Verification items for the finished model (mm, model axes). A direction names the side the tool comes from. Coordinates: 2 decimals unless noted, no trailing zeros. Loops run counter-clockwise (first coordinate to the right, second up) from the corner with the lowest first, then second, coordinate; pieces in that order, holes last. Notation, with made-up numbers: (48.5, -7.75) -> (55.5, -7.75) arc R15 cw to (55.5, 14.25) -> close; hole circle Ø5 at (69.5, 57). An arc over 180 degrees is marked (long way). Answer as a JSON object with one key per item and string values. Group by question number.
Q1. Gauge pin test, flat ends, axial feed: pin 1 Ø1.5 at (x, y) = (11, 10.5) entering from -Z; pin 2 Ø1.5 at (x, z) = (8, -28.5) entering from -Y; pin 3 Ø1.5 at (y, z) = (7.5, -29) entering from +X. Record the tip position at first contact, or that the pin passes through.
Q2. Release check for a two-part mould opening along X. For faces 1 (the cylindrical face through (-0.53, 13.82, -28.87)), 2 (the flat face through (-1, 0, 0)), 3 (the cylindrical face through (-0.53, -13.82, -28.74)), 4 (the flat face through (37.744, 0, -29)) record: released by +X, released by -X, zero draft, split by the parting line, or undercut.
Q3. Cross-section at D-D on y = 15. Record the boundary of the cut face in (x, z) (3 decimals), and give its area (3 significant figures).
Q4. Cross-section at B-B on y = 5. Record the boundary of the cut face in (x, z) (3 decimals).
Q5. Cross-section at A-A on x = 18.5. Record the boundary of the cut face in (y, z).
Q6. Set-up check for faces 5 (the flat face through (-3, -18, -31.75)), 6 (the flat face through (34.2, -6.47, -0.73)), 7 (the flat face through (-1, 16.764, -13)), 8 (the flat face through (-33.096, 0, -1)): record each of +Z, -Z, +X, -X, +Y, -Y from which the full face is reachable in a straight line by a thin tool's end or side.
Q7. Scan lines: L1, parallel to Y at x = 14, z = -24; L2, parallel to X at y = 0, z = -24; L3, parallel to Z at x = -35, y = 9. Record each from-to range of solid material in increasing order.
Q8. Cross-section at C-C on z = -6.5. Record the boundary of the cut face in (x, y).
```python
from build123d import *

# Parameters (mm, degrees)
F0_W      = 79.0448
F0_H      = 37.211
F0_W_2    = 75.438
F0_H_2    = 33.528
F1_DEPTH  = 31.75
F0_W_3    = 29.9212
F0_H_3    = 22.098
F2_DEPTH  = 1.4732
F5_DEPTH  = 35.3695
F7_DEPTH  = 77.2414
F8_W      = 1.778
F8_H      = 2.9464
F9_DEPTH  = 37.211
F10_W     = 1.778
F10_H     = 2.9464
F11_DEPTH = 75.4888


with BuildPart() as f1:
    # F0 (on Top) → F1 (new body)
    with BuildSketch(Plane.XY):
        Rectangle(F0_W, F0_H)
        Rectangle(F0_W_2, F0_H_2, mode=Mode.SUBTRACT)
    extrude(amount=-F1_DEPTH)

    # F0 (on Top) → F2 (join)
    with BuildSketch(Plane.XY):
        Rectangle(F0_W_2, F0_H_2)
        with Locations((-18.1356, 0)):
            Rectangle(F0_W_3, F0_H_3, mode=Mode.SUBTRACT)
        Polygon((9.525, 9.0805), (36.449, 9.0805), (36.449, -3.07601), (31.877, -9.9695), (14.097, -9.9695), (9.525, -3.07601), align=None, mode=Mode.SUBTRACT)
    extrude(amount=-F2_DEPTH)

    # F4 (on face) → F5 (join, through all)
    with BuildSketch(Plane.XZ.offset(18.6055)):
        with BuildLine():
            Line((-37.719, -25.8572), (-37.719, -31.75))
            ThreePointArc((-37.719, -31.75), (-34.7726, -28.8036), (-37.719, -25.8572))
        make_face()
        with BuildLine():
            Line((37.719, -31.75), (37.719, -25.8572))
            ThreePointArc((37.719, -25.8572), (34.7726, -28.8036), (37.719, -31.75))
        make_face()
    extrude(amount=-F5_DEPTH)

    # F6 (on face) → F7 (join, through all)
    with BuildSketch(Plane(origin=(-39.5224, 0, 0), x_dir=(0, -1, 0), z_dir=(-1, 0, 0))):
        with BuildLine():
            Line((-16.764, -25.8572), (-16.764, -31.75))
            ThreePointArc((-16.764, -31.75), (-13.8176, -28.8036), (-16.764, -25.8572))
        make_face()
        with BuildLine():
            Line((16.764, -31.75), (16.764, -25.8572))
            ThreePointArc((16.764, -25.8572), (13.8176, -28.8036), (16.764, -31.75))
        make_face()
    extrude(amount=-F7_DEPTH)

    # F8 (on face) → F9 (cut, through all)
    with BuildSketch(Plane.XZ.offset(18.6055)):
        with Locations((-38.6334, -28.8036)):
            Rectangle(F8_W, F8_H)
        with Locations((38.6334, -28.8036)):
            Rectangle(F8_W, F8_H)
    extrude(amount=-F9_DEPTH, mode=Mode.SUBTRACT)

    # F10 (on face) → F11 (cut, through all)
    with BuildSketch(Plane(origin=(-37.7444, 0, 0), x_dir=(0, -1, 0), z_dir=(-1, 0, 0))):
        with Locations((-17.7165, -28.8036)):
            Rectangle(F10_W, F10_H)
        with Locations((17.7165, -28.8036)):
            Rectangle(F10_W, F10_H)
    extrude(amount=-F11_DEPTH, mode=Mode.SUBTRACT)


solid = f1.part
```
Computed values:
{
 "1": {"pin 1": "stops at z = -1.47", "pin 2": "stops at y = -16.83", "pin 3": "stops at x = 37.74"},
 "2": {"face 1": "undercut", "face 2": "zero draft", "face 3": "undercut", "face 4": "released by +X"},
 "3": {"outline": "(-39.522, -31.75) -> (-37.719, -31.75) arc R2.946 ccw to (-35.955, -31.164) -> (35.955, -31.164) arc R2.946 ccw to (37.719, -31.75) -> (39.522, -31.75) -> (39.522, -30.277) -> (37.744, -30.277) -> (37.744, -27.33) -> (39.522, -27.33) -> (39.522, 0) -> (-39.522, 0) -> (-39.522, -27.33) -> (-37.744, -27.33) -> (-37.744, -30.277) -> (-39.522, -30.277) -> close; hole (-37.719, -25.857) arc R2.946 cw to (-35.955, -26.444) -> (35.955, -26.444) arc R2.946 cw to (37.719, -25.857) -> (37.719, -1.473) -> (-37.719, -1.473) -> close", "area": "574 mm²"},
 "4": {"outline": "(-39.522, -31.75) -> (-37.719, -31.75) arc R2.946 ccw to (-37.719, -25.857) -> (-37.719, -1.473) -> (-33.096, -1.473) -> (-33.096, 0) -> (-39.522, 0) -> (-39.522, -27.33) -> (-37.744, -27.33) -> (-37.744, -30.277) -> (-39.522, -30.277) -> close; (-3.175, -1.473) -> (9.525, -1.473) -> (9.525, 0) -> (-3.175, 0) -> close; (36.449, -1.473) -> (37.719, -1.473) -> (37.719, -25.857) arc R2.946 ccw to (37.719, -31.75) -> (39.522, -31.75) -> (39.522, -30.277) -> (37.744, -30.277) -> (37.744, -27.33) -> (39.522, -27.33) -> (39.522, 0) -> (36.449, 0) -> close"},
 "5": {"outline": "(-18.61, -31.75) -> (-16.76, -31.75) arc R2.95 ccw to (-16.76, -25.86) -> (-16.76, -1.47) -> (-9.97, -1.47) -> (-9.97, 0) -> (-18.61, 0) -> (-18.61, -27.33) -> (-16.83, -27.33) -> (-16.83, -30.28) -> (-18.61, -30.28) -> close; (9.08, -1.47) -> (16.76, -1.47) -> (16.76, -25.86) arc R2.95 ccw to (16.76, -31.75) -> (18.61, -31.75) -> (18.61, -30.28) -> (16.83, -30.28) -> (16.83, -27.33) -> (18.61, -27.33) -> (18.61, 0) -> (9.08, 0) -> close"},
 "6": {"face 5": "-Z, +X, -X, +Y, -Y", "face 6": "+Z", "face 7": "none", "face 8": "+Z, -Z"},
 "7": {"L1": "y = -18.61 to -16.76, 16.76 to 18.61", "L2": "x = -39.52 to -37.72, 37.72 to 39.52", "L3": "z = -29.94 to -27.67, -1.47 to 0"},
 "8": {"outline": "(-39.52, -18.61) -> (39.52, -18.61) -> (39.52, 18.61) -> (-39.52, 18.61) -> close; hole (-37.72, -16.76) -> (37.72, -16.76) -> (37.72, 16.76) -> (-37.72, 16.76) -> close"}
}
